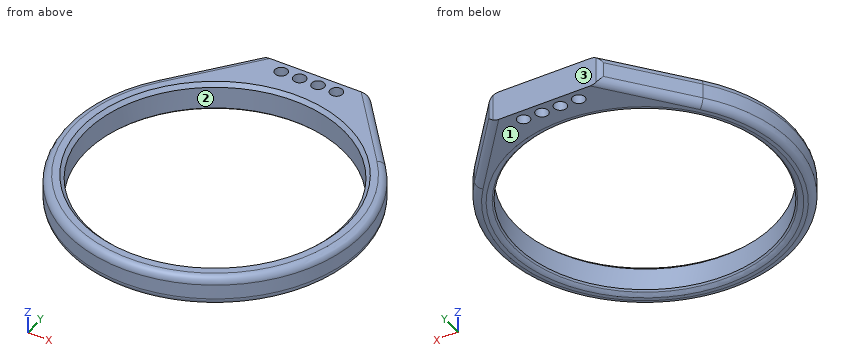
```python
from build123d import *

# Parameters (mm, degrees)
SKETCH1_R                = 35.1
BOSS_EXTRUDE1_DEPTH      = 8
M3_CLEARANCE_HOLE1_D     = 3.4
M3_CLEARANCE_HOLE1_DEPTH = 8
M3_CLEARANCE_HOLE1_TIP   = 1.021463052
CHAMFER1_SIZE            = 1
FILLET1_R                = 2


with BuildPart() as part:
    # Sketch1 → Boss-Extrude1 (new body)
    with BuildSketch(Plane.XY):
        with BuildLine():
            Line((-15, 45), (0, 45))
            Line((0, 45), (15, 45))
            Line((15, 45), (31.062744721, 25.201307315))
            ThreePointArc((31.062744721, 25.201307315), (0, -40), (-31.062744721, 25.201307315))
            Line((-31.062744721, 25.201307315), (-15, 45))
        make_face()
        Circle(SKETCH1_R, mode=Mode.SUBTRACT)
    extrude(amount=BOSS_EXTRUDE1_DEPTH)

    # M3 Clearance Hole1
    with Locations(Plane.XY.offset(8)):
        with Locations((7.5, 42), (-2.5, 42), (-7.5, 42), (2.5, 42)):
            Hole(M3_CLEARANCE_HOLE1_D / 2, depth=M3_CLEARANCE_HOLE1_DEPTH)
            with Locations((0, 0, -(M3_CLEARANCE_HOLE1_DEPTH + M3_CLEARANCE_HOLE1_TIP / 2))):  # 118° drill point
                Cone(0, M3_CLEARANCE_HOLE1_D / 2, M3_CLEARANCE_HOLE1_TIP, mode=Mode.SUBTRACT)

    # Chamfer1
    chamfer1_edges = [part.edges().sort_by_distance(p)[0] for p in [
        (-35.1, 0, 0),
        (-35.1, 0, 8),
    ]]
    chamfer(chamfer1_edges, length=CHAMFER1_SIZE)

    # Fillet1
    fillet1_edges = [part.edges().sort_by_distance(p)[0] for p in [
        (23.031372361, 35.100653658, 8),
        (-36.1, 0, 0),
        (-23.031372361, 35.100653658, 8),
        (23.031372361, 35.100653658, 0),
        (0, -40, 0),
        (-23.031372361, 35.100653658, 0),
        (0, -40, 8),
        (-15, 45, 4),
        (15, 45, 4),
    ]]
    fillet(fillet1_edges, radius=FILLET1_R)


solid = part.part
```
Here's how the part is built. I have some questions about the finished solid (model axes, mm). Face numbers are marked on the shaded views. Give positions to 0.01 mm unless a question says otherwise; leave off trailing zeros. Write each loop counter-clockwise with the first axis right and the second up, starting at its lowest first coordinate (ties: lowest second). Pieces come first, ordered by that corner, then holes.
(1) Will these pins go through, and if not, where does the flat tip stop? pin 1 (1 mm diameter, centred on y = 30, z = 5.5, fed in from +X); pin 2 (2.5 mm diameter, centred on x = 7.5, y = 42, fed in from +Z); pin 3 (4.5 mm diameter, centred on x = 2.5, y = 42, fed in from -Z); pin 4 (4 mm diameter, centred on x = 24, z = 1, fed in from -Y).
Output values:
pin 1: stops at x = 27.58
pin 2: passes through
pin 3: stops at z = 0
pin 4: stops at y = -33.3
(2) Thinking about a two-plate mould opening in Y: for the marked faces 1, 2 and 3, which applies, pulls with the +Y half, pulls with the -Y half, needs draft (parallel to the pull), parting line crosses it, or undercut?
Output values:
face 1: needs draft
face 2: undercut
face 3: pulls with the +Y half
(3) Imagine slicing it at B-B, the plane x = -8. Count the separate pieces of the cut face and the enclosed holes in it, and give its area (3 significant figures).
Output values:
separate pieces: 3
enclosed holes: 0
area: 96.7 mm2
(4) If I drill on L1, parallel to Y at x = 0, z = 2.55; L2, parallel to X at y = 42, z = 3.25; L3, parallel to Y at x = -2.5, z = 3.75, over which ranges is the centre line in solid material (lowest first)?
Output values:
L1: y = -40 to -35.1, 35.1 to 45
L2: x = -17.43 to -9.2, -5.8 to -4.2, -0.8 to 0.8, 4.2 to 5.8, 9.2 to 17.43
L3: y = -39.92 to -35.01, 35.01 to 40.3, 43.7 to 45
(5) Imagine slicing it at A-A, the plane z = 3. Write out the boundary of the cut face in (x, y).
Output values:
outline: (-31.06, 25.2) arc R40 ccw (long way) to (31.06, 25.2) - (15.6, 44.26) arc R2 ccw to (14.05, 45) - (-14.05, 45) arc R2 ccw to (-15.6, 44.26) - close; hole circle Ø70.2 at (0, 0); hole circle Ø3.4 at (-7.5, 42); hole circle Ø3.4 at (-2.5, 42); hole circle Ø3.4 at (2.5, 42); hole circle Ø3.4 at (7.5, 42)
